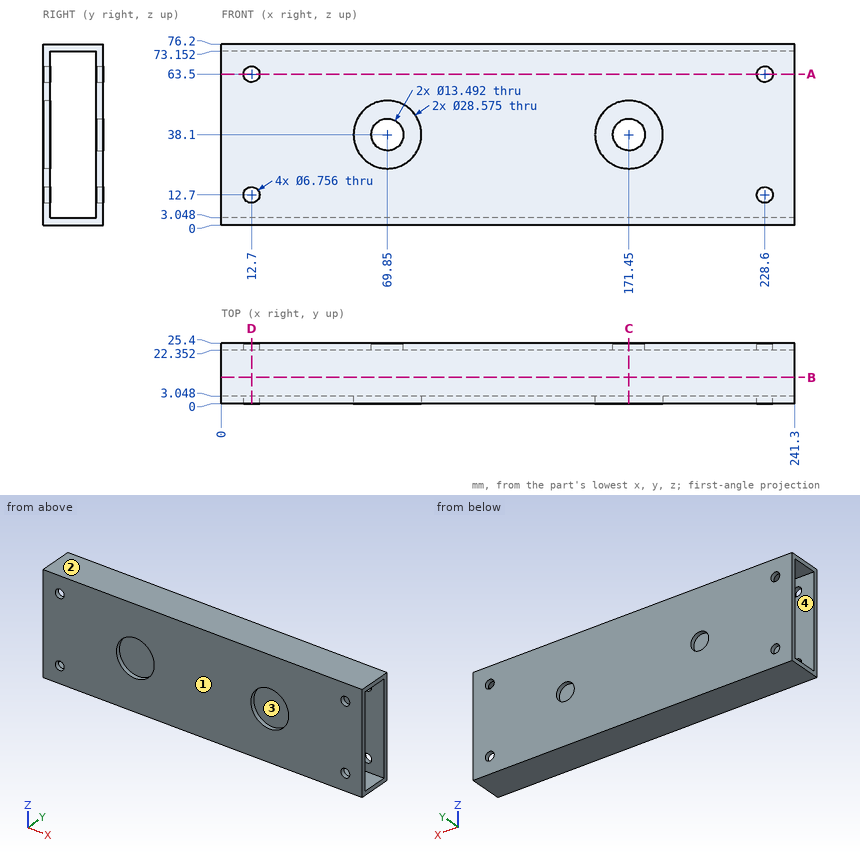
Part print with two shaded views. Sizes in mm from the minimum x, y, z corner. Give positions to 0.01 mm unless a question says otherwise; leave off trailing zeros. Order: outer loops, then holes, each group sorted by start corner. A loop starts at its lowest first (then second) coordinate and runs counter-clockwise, first axis right, second up.
(1) Flat gauge pin, fed straight in: pin 1 (8 mm diameter, centred on x = 12.7, z = 63.5, fed in from -Y). Where does the tip first touch, or does it go through?
(2) Drill centre lines: L1, parallel to X at y = 1.5, z = 38.1; L2, parallel to X at y = 23, z = 63.5; L3, parallel to Z at x = 228.6, y = 1.65. Where is each one in solid material? Low to high.
(3) Mould opens along Z. For the marked faces 1, 2, 3 and 4 say: released by +Z, released by -Z, zero draft, split by the parting line, or undercut.
(4) Saw through at B-B, the plane y = 11. Give the cut face in (x, z).
(5) Saw through at C-C, the plane x = 171.45. Give the cut face in (y, z).
(6) Saw through at A-A, the plane z = 63.5. Give the cut face in (x, y), then the cut area to 3 significant figures.
(7) Saw through at D-D, the plane x = 12.7. Give the cut face in (y, z).
Results found:
1. pin 1: stops at y = 0
2. L1: x = 0 to 55.56, 84.14 to 157.16, 185.74 to 241.3
2. L2: x = 0 to 9.32, 16.08 to 225.22, 231.98 to 241.3
2. L3: z = 0 to 9.32, 16.08 to 60.12, 66.88 to 76.2
3. face 1: zero draft
3. face 2: released by +Z
3. face 3: undercut
3. face 4: undercut
4. outline: (0, 0) - (241.3, 0) - (241.3, 3.05) - (0, 3.05) - close; (0, 73.15) - (241.3, 73.15) - (241.3, 76.2) - (0, 76.2) - close
5. outline: (0, 0) - (25.4, 0) - (25.4, 31.35) - (22.35, 31.35) - (22.35, 3.05) - (3.05, 3.05) - (3.05, 23.81) - (0, 23.81) - close; (0, 52.39) - (3.05, 52.39) - (3.05, 73.15) - (22.35, 73.15) - (22.35, 44.85) - (25.4, 44.85) - (25.4, 76.2) - (0, 76.2) - close
6. outline: (0, 0) - (9.32, 0) - (9.32, 3.05) - (0, 3.05) - close; (0, 22.35) - (9.32, 22.35) - (9.32, 25.4) - (0, 25.4) - close; (16.08, 0) - (225.22, 0) - (225.22, 3.05) - (16.08, 3.05) - close; (16.08, 22.35) - (225.22, 22.35) - (225.22, 25.4) - (16.08, 25.4) - close; (231.98, 0) - (241.3, 0) - (241.3, 3.05) - (231.98, 3.05) - close; (231.98, 22.35) - (241.3, 22.35) - (241.3, 25.4) - (231.98, 25.4) - close
6. area: 1,390 mm2
7. outline: (0, 0) - (25.4, 0) - (25.4, 9.32) - (22.35, 9.32) - (22.35, 3.05) - (3.05, 3.05) - (3.05, 9.32) - (0, 9.32) - close; (0, 16.08) - (3.05, 16.08) - (3.05, 60.12) - (0, 60.12) - close; (0, 66.88) - (3.05, 66.88) - (3.05, 73.15) - (22.35, 73.15) - (22.35, 66.88) - (25.4, 66.88) - (25.4, 76.2) - (0, 76.2) - close; (22.35, 16.08) - (25.4, 16.08) - (25.4, 60.12) - (22.35, 60.12) - close
